Geometry: final body of the model. Coordinates: model frame, mm. Round coordinates to 2 decimals unless told otherwise and drop trailing zeros. Loops run counter-clockwise (first coordinate to the right, second up) from the corner with the lowest first, then second, coordinate; pieces in that order, holes last. Notation, with made-up numbers: M 87.5,59 L 126.5,59 A25 ccw 126.5,77 Z; hole C 81.5,-0.5 d3. An arc over 180 degrees is marked long. Answer as a JSON object with one key per item and string values.
```python
from build123d import *

# Parameters (mm, degrees)
F0_R     = 11.2
F1_DEPTH = 7


with BuildPart() as f1:
    # F0 (on Top) → F1 (new body)
    with BuildSketch(Plane.XY):
        with BuildLine():
            ThreePointArc((0.629275, 42.658791), (-0.007055, 43.079038), (-0.634205, 42.645211))
            Line((-0.634205, 42.645211), (-0.644867, 42.615845))
            Line((-0.644867, 42.615845), (-10.810192, 14.617693))
            ThreePointArc((-10.810192, 14.617693), (-9.723034, 9.72304), (-14.617687, 10.810197))
            Line((-14.617687, 10.810197), (-42.658791, 0.629275))
            ThreePointArc((-42.658791, 0.629275), (-43.079038, -0.007039), (-42.64524, -0.634194))
            Line((-42.64524, -0.634194), (-42.615845, -0.644866))
            Line((-42.615845, -0.644866), (-14.617691, -10.810185))
            ThreePointArc((-14.617691, -10.810185), (-9.723041, -9.723034), (-10.810191, -14.617685))
            Line((-10.810191, -14.617685), (-0.629275, -42.658791))
            ThreePointArc((-0.629275, -42.658791), (0.007037, -43.079038), (0.634193, -42.645243))
            Line((0.634193, -42.645243), (0.644866, -42.615845))
            Line((0.644866, -42.615845), (10.810179, -14.617689))
            ThreePointArc((10.810179, -14.617689), (9.723034, -9.72304), (14.617682, -10.810185))
            Line((14.617682, -10.810185), (42.658791, -0.629275))
            ThreePointArc((42.658791, -0.629275), (43.079038, 0.007064), (42.645194, 0.634212))
            Line((42.645194, 0.634212), (42.615845, 0.644868))
            Line((42.615845, 0.644868), (14.617696, 10.810198))
            ThreePointArc((14.617696, 10.810198), (9.72304, 9.723034), (10.810204, 14.617689))
            Line((10.810204, 14.617689), (0.629275, 42.658791))
        make_face()
        Circle(F0_R, mode=Mode.SUBTRACT)
    extrude(amount=F1_DEPTH)


solid = f1.part
```
1) Line query: probe 1 along Y at (x, z) = (0, 2); probe 2 along Y at (x, z) = (-20, 2.25); probe 3 along Y at (x, z) = (-20.5, 3.25). Output: solid intervals per line, ascending.
Geometry results:
{"probe 1": "-43.08 to -11.2, 11.2 to 43.08", "probe 2": "-8.86 to 8.86", "probe 3": "-8.67 to 8.67"}
2) Cut plane C-C on y = -7. Return the cut outline in (x, z), and give its area (3 significant figures).
Geometry results:
{"outline": "M -25.11,0 L -8.74,0 L -8.74,7 L -25.11,7 Z; M 8.74,0 L 25.11,0 L 25.11,7 L 8.74,7 Z", "area": "229 mm2"}
3) Cut plane A-A on x = -4. Return the cut outline in (y, z), and give its area (3 significant figures).
Geometry results:
{"outline": "M -33.37,0 L -10.46,0 L -10.46,7 L -33.37,7 Z; M 10.46,0 L 33.37,0 L 33.37,7 L 10.46,7 Z", "area": "321 mm2"}
4) Cut plane D-D on x = 31. Return the cut outline in (y, z).
Geometry results:
{"outline": "M -4.86,0 L 4.86,0 L 4.86,7 L -4.86,7 Z"}
5) First-contact query: pin 1 (1.5 mm diameter, centred on x = 13.5, z = 5, fed in from +Y); pin 2 (1.5 mm diameter, centred on x = -0.5, z = 2.5, fed in from +Y); pin 3 (2 mm diameter, centred on x = -20, z = 5, fed in from -Y). Flat tips, straight axial feed; report the tip coordinate or a pass-through.
Geometry results:
{"pin 1": "y = 10.11", "pin 2": "y = 43.08", "pin 3": "y = -9.22"}
6) Pull-direction query (Y, two-part tool) for faces 1 (the face through (9.665, -9.783, 3.451)), 2 (the face through (-7, 10, 0)), 3 (the face through (5.79, 28.44, 3.45)), 4 (the face through (9.783, 9.665, 3.451)); classes: +Y half, -Y half, draft (parallel to the pull), parting line (faces both ways), or undercut.
Geometry results:
{"face 1": "undercut", "face 2": "draft", "face 3": "+Y half", "face 4": "undercut"}
